from build123d import *

# Parameters (mm, degrees)
F1_DEPTH  = 13.6
F3_D      = 5.1
F5_DEPTH  = 12
F6_DEPTH  = 25
F7_DEPTH  = 15
F8_D      = 5.1
F9_W      = 5.1
F9_H      = 5.7
F10_DEPTH = 25
F4_W      = 6.8
F4_H      = 4
F11_DEPTH = 25


# Not quite as in the source:
# - a feature names something its author has since deleted; it is built from what else it names


with BuildPart() as f1:
    # F0 (on Right) → F1 (new body)
    with BuildSketch(Plane.YZ):
        Polygon((-70, 0), (0, 0), (-60, 135), (-70, 135), align=None)
    extrude(amount=F1_DEPTH)

    # F3 (through all)
    with Locations(Plane.XZ.offset(70)):
        with Locations((6.8, 15), (6.8, 120)):
            Hole(F3_D / 2)

    # F4 (on face) → F5 (cut)
    with BuildSketch(Plane(origin=(0, 0, 0), x_dir=(1, 0, 0), z_dir=(0, 0, -1))):
        with BuildLine():
            ThreePointArc((9.35, 55), (8.603122292, 56.803122292), (6.8, 57.55))
            Line((6.8, 57.55), (6.8, 55))
            Line((6.8, 55), (6.8, 52.45))
            ThreePointArc((6.8, 52.45), (8.603122292, 53.196877708), (9.35, 55))
        make_face()
        with BuildLine():
            ThreePointArc((9.35, 15), (8.603122292, 16.803122292), (6.8, 17.55))
            ThreePointArc((6.8, 17.55), (4.996877708, 13.196877708), (9.35, 15))
        make_face()
        with BuildLine():
            Line((6.8, 55), (6.8, 57.55))
            ThreePointArc((6.8, 57.55), (4.25, 55), (6.8, 52.45))
            Line((6.8, 52.45), (6.8, 55))
        make_face()
    extrude(amount=-F5_DEPTH, mode=Mode.SUBTRACT)

    # F2 (on face) → F6 (join)
    with BuildSketch(Plane.XZ.offset(70)):
        Polygon((11.9, 122.9444863729), (6.8, 125.8889727457), (1.7, 122.9444863729), (1.7, 117.0555136271), (6.8, 114.1110272543), (11.9, 117.0555136271), align=None)
    extrude(amount=-F6_DEPTH)

    # F7 (cut): a face of the model
    f7_faces = [f1.faces().sort_by_distance(p)[0] for p in [
        (6.8, -45, 120),
    ]]
    extrude(f7_faces, amount=-F7_DEPTH, mode=Mode.SUBTRACT)

    # F8 (through all)
    with Locations(Plane.XZ.offset(70)):
        with Locations((6.8, 120)):
            Hole(F8_D / 2)

    # F9 (on face) → F10 (cut)
    with BuildSketch(Plane(origin=(0, 0, 0), x_dir=(0, -1, 0), z_dir=(-1, 0, 0))):
        with Locations((12.45, 7.15)):
            Rectangle(F9_W, F9_H)
        with Locations((17.55, 7.15)):
            Rectangle(F9_W, F9_H)
    extrude(amount=-F10_DEPTH, mode=Mode.SUBTRACT)

    # F4 (on face) → F11 (cut)
    with BuildSketch(Plane(origin=(0, 0, 0), x_dir=(1, 0, 0), z_dir=(0, 0, -1))):
        with Locations((10.2, 2)):
            Rectangle(F4_W, F4_H)
        with Locations((3.4, 2)):
            Rectangle(F4_W, F4_H)
    extrude(amount=-F11_DEPTH, mode=Mode.SUBTRACT)


solid = f1.part
The listing builds one solid part. Answer for the finished solid, in the listing's coordinates (mm). A direction names the side the tool comes from. Give positions to 0.01 mm unless a question says otherwise; leave off trailing zeros. Loops run counter-clockwise (first coordinate to the right, second up) from the corner with the lowest first, then second, coordinate; pieces in that order, holes last.
Item 1: A cutting plane is placed at C-C (x = 3). Give the vertices of the cut face in (y, z).
Derived:
outline: (-70, 0) - (-4, 0) - (-4, 9) - (-51.69, 116.3) - (-60, 116.3) - (-60, 123.7) - (-54.98, 123.7) - (-60, 135) - (-70, 135) - close; hole (-20.1, 4.3) - (-9.9, 4.3) - (-9.9, 10) - (-20.1, 10) - close
Item 2: Determine the mould class of faces 1 (the flat face through (13.6, -45, 53)), 2 (the flat face through (5.2, -17.2, 4.3)), 3 (the cylindrical face through (7.13, -64.93, 122.53)), 4 (the flat face through (0, -45, 53)) for opening direction X: +X half, -X half, draft (parallel to the pull), parting line (faces both ways), or undercut.
Derived:
face 1: +X half
face 2: draft
face 3: undercut
face 4: -X half
Item 3: A cutting plane is placed at B-B (z = 15). Give the vertices of the cut face in (x, y), then the cut area to 3 significant figures.
Derived:
outline: (0, -70) - (4.25, -70) - (4.25, -6.67) - (0, -6.67) - close; (9.35, -70) - (13.6, -70) - (13.6, -6.67) - (9.35, -6.67) - close
area: 538 mm2
Item 4: Each of these flat-tipped pins is pushed along its axis until it touches: pin 1 Ø6.5 at (x, y) = (6.8, -15) entering from +Z; pin 2 Ø1 at (x, y) = (5, -22) entering from +Z (3 decimals); pin 3 Ø3 at (x, y) = (9, -17) entering from +Z (3 decimals); pin 4 Ø4.5 at (x, z) = (6.8, 15) entering from +Y. Where does it stop, or does it pass through?
Derived:
pin 1: stops at z = 41.06
pin 2: stops at z = 50.625
pin 3: stops at z = 41.625
pin 4: passes through
Item 5: A cutting plane is placed at A-A (y = -36). Give the vertices of the cut face in (x, z).
Derived:
outline: (0, 0) - (13.6, 0) - (13.6, 81) - (0, 81) - close; hole circle Ø5.1 at (6.8, 15)
Item 6: A cutting plane is placed at D-D (z = 90). Give the vertices of the cut face in (x, y).
Derived:
outline: (0, -70) - (13.6, -70) - (13.6, -40) - (0, -40) - close
Item 7: A tool of negligible diameter and unlimited length cuts with its end or side. For faces 5 (the flat face through (7, -4, 4)), 6 (the flat face through (1.7, -57, 120)), 7 (the flat face through (7, -37, 0)), 8 (the flat face through (7, -9.9, 7)), 9 (the flat face through (7, -15, 12)), from which of +Z, -Z, +X, -X, +Y, -Y can it reach the whole face along a straight path? Write none if from no direction.
Derived:
face 5: +Z, -Z, +X, -X, +Y
face 6: +Y
face 7: -Z, +X, -X, +Y, -Y
face 8: +X, -X
face 9: -Z
Item 8: Find the intervals of material crossed by line 1 along Y through (x, z) = (1, 7); line 2 along Y through (x, z) = (6.8, 11.6); line 3 along Z through (x, y) = (9, -12), in increasing order.
Derived:
line 1: y = -70 to -20.1, -9.9 to -4
line 2: y = -70 to -57.55, -52.45 to -17.55, -12.45 to -5.16
line 3: z = 0 to 4.3, 10 to 13.71, 16.29 to 27
